Design review of the part shown in the three views and the two pictorial views. Dimensions are in mm from the part's minimum x, y and z. Coordinates: 2 decimals unless noted, no trailing zeros. Write each loop counter-clockwise with the first axis right and the second up, starting at its lowest first coordinate (ties: lowest second). Pieces come first, ordered by that corner, then holes.
Q1. Take a section at C-C, the plane y = 0.9. State how many separate pieces and enclosed holes the cut face has, plus the area to 3 significant figures.
Q2. For L1, parallel to Z at x = 49, y = 1.9; L2, parallel to Z at x = 8, y = 0.65; L3, parallel to Z at x = 35.5, y = 2.2 (1 decimal), list the stretches that pass through material, from the lowest coordinate up.
Q3. Take a section at A-A, the plane x = 58.5. Write out the cut boundary in (y, z) (1 decimal), plus the area to 3 significant figures.
Q4. For pin 1 Ø1 at (x, y) = (49, 2.5) entering from +Z, flat-tipped, find the tip position at first contact; note if it passes through.
Q5. Take a section at B-B, the plane z = 38.5. Write out the cut boundary in (x, y) (1 decimal).
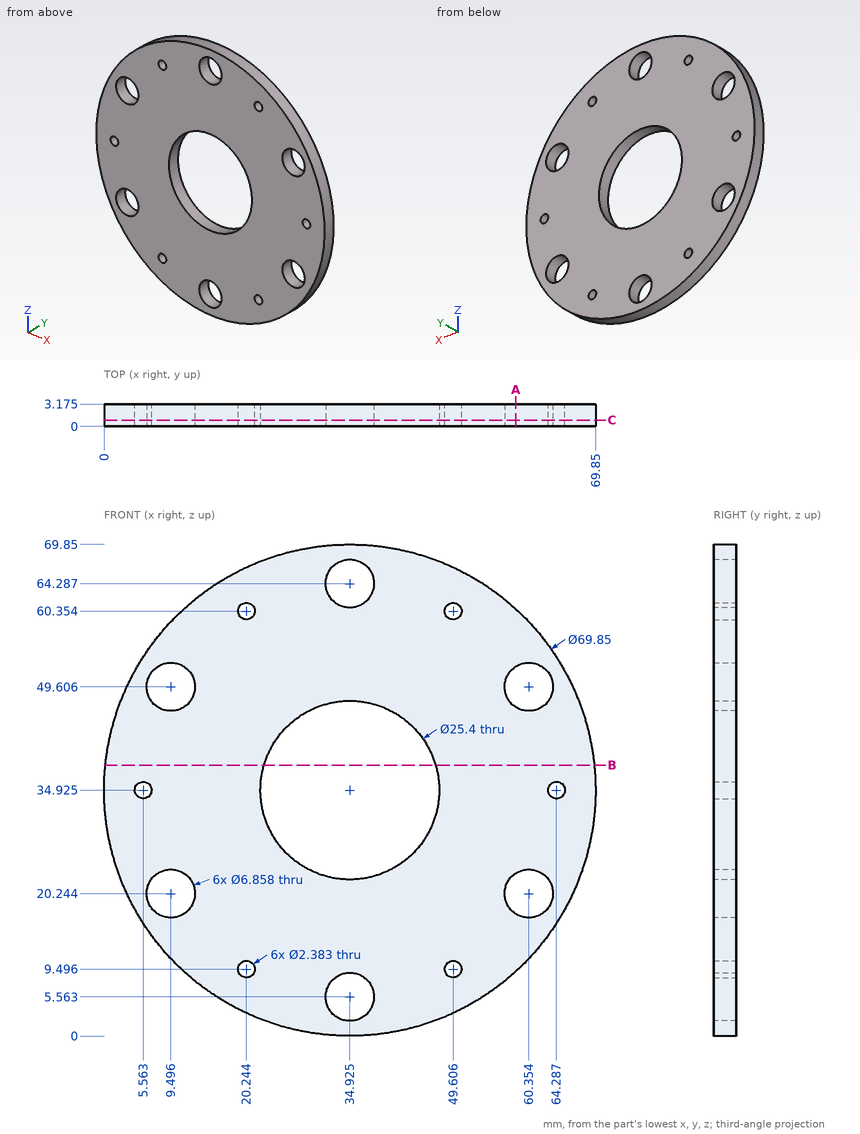
Responses:
1. separate pieces: 1
1. enclosed holes: 13
1. area: 3,080 mm2
2. L1: z = 2.96 to 8.47, 10.52 to 59.33, 61.38 to 66.89
2. L2: z = 12.68 to 17.16, 23.33 to 46.52, 52.69 to 57.17
2. L3: z = 0 to 2.2, 8.9 to 22.2, 47.6 to 60.9, 67.7 to 69.8
3. outline: (0, 9.2) - (3.2, 9.2) - (3.2, 17.4) - (0, 17.4) - close; (0, 23.1) - (3.2, 23.1) - (3.2, 46.7) - (0, 46.7) - close; (0, 52.5) - (3.2, 52.5) - (3.2, 60.7) - (0, 60.7) - close
3. area: 127 mm2
4. pin 1: stops at z = 67.1
5. outline: (0.2, 0) - (22.7, 0) - (22.7, 3.2) - (0.2, 3.2) - close; (47.1, 0) - (69.7, 0) - (69.7, 3.2) - (47.1, 3.2) - close
